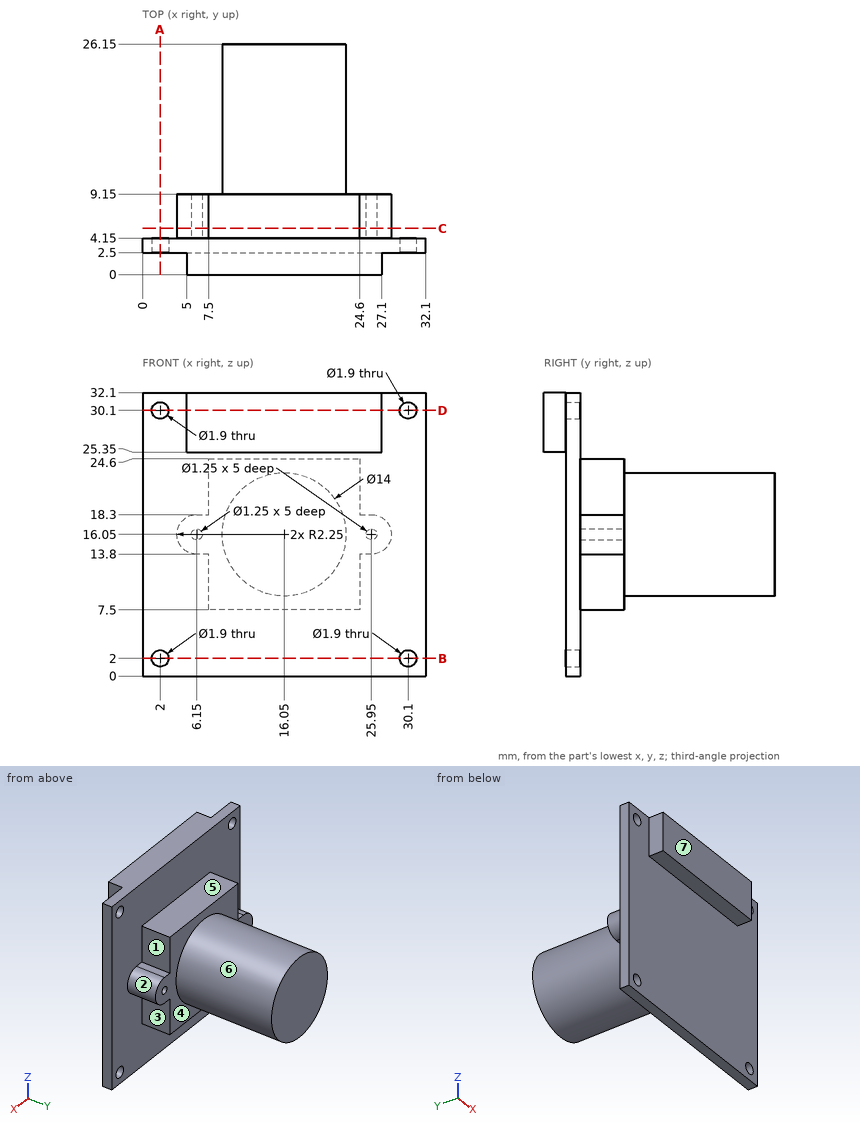
The drawing under review shows one solid part. Ordinate dimensions are in mm from its lowest x, y, z. A direction names the side the tool comes from. Coordinates: 2 decimals unless noted, no trailing zeros. Loops run counter-clockwise (first coordinate to the right, second up) from the corner with the lowest first, then second, coordinate; pieces in that order, holes last.
Item 1: Add section C-C (y = 5.25). Write out the cut boundary in (x, z) (3 decimals).
Completed:
outline: (6.15, 13.8) - (7.5, 13.8) - (7.5, 7.5) - (24.6, 7.5) - (24.6, 13.8) - (25.95, 13.8) arc R2.25 ccw to (25.95, 18.3) - (24.6, 18.3) - (24.6, 24.6) - (7.5, 24.6) - (7.5, 18.3) - (6.15, 18.3) arc R2.25 ccw to start; hole circle Ø1.25 at (6.15, 16.05); hole circle Ø1.25 at (25.95, 16.05)
Item 2: Clearance check with flat-ended pins moving along their axes: pin 1 (1.5 mm diameter, centred on x = 15.5, y = 16.5, fed in from +Z); pin 2 (1 mm diameter, centred on x = 25.95, z = 16.05, fed in from -Y); pin 3 (1.7 mm diameter, centred on x = 30.1, z = 2, fed in from -Y); pin 4 (5 mm diameter, centred on x = 17, z = 28, fed in from +Y). State where each tip first meets the part, or that it passes through.
Completed:
pin 1: stops at z = 23.05
pin 2: stops at y = 2.5
pin 3: passes through
pin 4: stops at y = 4.15
Item 3: For the marked faces 1, 2, 3 and 4, list the 3-axis set-ups (+Z, -Z, +X, -X, +Y, -Y) from which the entire face can be reached by the end or side of a thin tool; tool diameter is ignored.
Completed:
face 1: +Z, +X, +Y
face 2: +X, +Y
face 3: -Z, +X, +Y
face 4: +Y
Item 4: Add section B-B (z = 2). Write out the cut boundary in (x, y), and give its area (3 significant figures).
Completed:
outline: (0, 2.5) - (1.05, 2.5) - (1.05, 4.15) - (0, 4.15) - close; (2.95, 2.5) - (29.15, 2.5) - (29.15, 4.15) - (2.95, 4.15) - close; (31.05, 2.5) - (32.1, 2.5) - (32.1, 4.15) - (31.05, 4.15) - close
area: 46.7 mm2
Item 5: Draft analysis for pull direction Z (two halves, no side actions). For the marked faces 5, 6 and 7, state which applies: pulls with the +Z half, pulls with the -Z half, needs draft (parallel to the pull), parting line crosses it, or undercut.
Completed:
face 5: pulls with the +Z half
face 6: parting line crosses it
face 7: needs draft
Item 6: Wall thickness on L1, parallel to X at y = 5.85, z = 16.05 (3 decimals); L2, parallel to Z at x = 6.15, y = 7.95 (3 decimals); L3, parallel to X at y = 3, z = 30.5: over which ranges is each line inside the solid? List them lowest first.
Completed:
L1: x = 3.9 to 5.525, 6.775 to 25.325, 26.575 to 28.2
L2: z = 13.8 to 15.425, 16.675 to 18.3
L3: x = 0 to 1.14, 2.86 to 29.24, 30.96 to 32.1
Item 7: Add section D-D (z = 30.1). Write out the cut boundary in (x, y).
Completed:
outline: (0, 2.5) - (1.05, 2.5) - (1.05, 4.15) - (0, 4.15) - close; (2.95, 2.5) - (5, 2.5) - (5, 0) - (27.1, 0) - (27.1, 2.5) - (29.15, 2.5) - (29.15, 4.15) - (2.95, 4.15) - close; (31.05, 2.5) - (32.1, 2.5) - (32.1, 4.15) - (31.05, 4.15) - close
Item 8: Add section A-A (x = 2). Write out the cut boundary in (y, z).
Completed:
outline: (2.5, 0) - (4.15, 0) - (4.15, 1.05) - (2.5, 1.05) - close; (2.5, 2.95) - (4.15, 2.95) - (4.15, 29.15) - (2.5, 29.15) - close; (2.5, 31.05) - (4.15, 31.05) - (4.15, 32.1) - (2.5, 32.1) - close
